Here's how the part is built. I have some questions about the finished solid (model axes, mm). A direction names the side the tool comes from. Give positions to 0.01 mm unless a question says otherwise; leave off trailing zeros. Write each loop counter-clockwise with the first axis right and the second up, starting at its lowest first coordinate (ties: lowest second). Pieces come first, ordered by that corner, then holes. Notation, with made-up numbers: (69.5, 80) -> (121.5, 80) arc R24 ccw to (121.5, 107) -> close; hole circle Ø5 at (24, 12.25). An arc over 180 degrees is marked (long way). Use CSV: the item, a comma, the result in double quotes. Start each with the question number.
(1) If we mould it in two halves opening along Y, with no side actions, what happens to faces 1 (the flat face through (60, 18, 8)), 2 (the flat face through (64, 18, 15))? For each: pulls with the +Y half, pulls with the -Y half, needs draft (parallel to the pull), parting line crosses it, or undercut.
(2) Suppose I cut it at C-C on z = 11.75. List the corners of the cut face in (x, y) for me, plus the area to 3 significant figures.
(3) Suppose I cut it at D-D on x = 9. List the corners of the cut face in (y, z) for me, plus the area to 3 significant figures.
(4) For pin 1 Ø4.5 at (x, y) = (31, 25.5) entering from +Z; pin 2 Ø2.5 at (x, y) = (3, 17.5) entering from +Z (1 decimal), each with a flat end and sliding along its axis, tell me the tip position at first contact or that it passes through.
(5) Suppose I cut it at A-A on x = 31. List the corners of the cut face in (y, z) for me.
(6) Suppose I cut it at B-B on y = 25.5. List the corners of the cut face in (x, z) for me (3 decimals).
(7) Which directions (+Z, -Z, +X, -X, +Y, -Y) give clear straight access to the entire face, cutting with the end or side of a thin tool? Please do faces 3 (the flat face through (31, 17, 0)), 4 (the flat face through (30, 2, 6)), 5 (the cylindrical face through (71, 3, 14)).
(8) I need wall thicknesses on L1, parallel to X at y = 19.5, z = 12.25; L2, parallel to X at y = 13.5, z = 8.25; L3, parallel to Y at x = 31, z = 2.35. Which ranges of each line are inside material? Lowest first, please. Write a range as [from, to].
from build123d import *

# Parameters (mm, degrees)
SKETCH_W             = 80
SKETCH_H             = 35
PAD_DEPTH            = 15
SKETCH001_R          = 2.5
POCKET_DEPTH         = 14
SKETCH002_W          = 61
SKETCH002_H          = 33.5
POCKET001_DEPTH      = 5
SKETCH003_R          = 1.5
POCKET002_DEPTH      = 5
SKETCH004_R          = 4
PAD001_DEPTH         = 5
SKETCH005_R          = 2
POCKET003_DEPTH      = 5
SKETCH006_W          = 16.25
SKETCH006_H          = 33
POCKET004_DEPTH      = 13
POCKET005_DEPTH      = 15.001
SKETCH008_R          = 2
POCKET006_DEPTH      = 5.001
POCKET006_DEPTH_BACK = -10.001
SKETCH009_R          = 2
POCKET007_DEPTH      = 2.75


with BuildPart() as part:
    # Sketch → Pad (new body)
    with BuildSketch(Plane.XY):
        with Locations((40, 17.5)):
            Rectangle(SKETCH_W, SKETCH_H)
    extrude(amount=PAD_DEPTH)

    # Sketch001 (on Face6 of Pad) → Pocket (cut)
    with BuildSketch(Plane.XY.offset(15)):
        with BuildLine():
            Line((2, 33), (60, 33))
            Line((60, 33), (60, 2))
            Line((53.5, 2), (60, 2))
            ThreePointArc((53.5, 2), (52, 6.5), (50.5, 2))
            Line((10.5, 2), (50.5, 2))
            ThreePointArc((10.5, 2), (9, 6.5), (7.5, 2))
            Line((2, 2), (7.5, 2))
            Line((2, 2), (2, 33))
        make_face()
        with Locations((9, 29)):
            Circle(SKETCH001_R, mode=Mode.SUBTRACT)
        with Locations((52, 29)):
            Circle(SKETCH001_R, mode=Mode.SUBTRACT)
    extrude(amount=-POCKET_DEPTH, mode=Mode.SUBTRACT)

    # Sketch002 (on Face5 of Pocket) → Pocket001 (cut)
    with BuildSketch(Plane.XY.offset(15)):
        with Locations((31.25, 17.5)):
            Rectangle(SKETCH002_W, SKETCH002_H)
    extrude(amount=-POCKET001_DEPTH, mode=Mode.SUBTRACT)

    # Sketch003 (on Face24 of Pocket001) → Pocket002 (cut)
    with BuildSketch(Plane.XY.offset(10)):
        with Locations((9, 29)):
            Circle(SKETCH003_R)
        with Locations((9, 4)):
            Circle(SKETCH003_R)
        with Locations((52, 29)):
            Circle(SKETCH003_R)
        with Locations((52, 4)):
            Circle(SKETCH003_R)
    extrude(amount=-POCKET002_DEPTH, mode=Mode.SUBTRACT)

    # Sketch004 (on Face4 of Pocket002) → Pad001 (join)
    with BuildSketch(Plane(origin=(0, 0, 0), x_dir=(1, 0, 0), z_dir=(0, 0, -1))):
        with Locations((31, -9.5)):
            Circle(SKETCH004_R)
        with Locations((31, -25.5)):
            Circle(SKETCH004_R)
    extrude(amount=-PAD001_DEPTH)

    # Sketch005 (on Face4 of Pad001) → Pocket003 (cut)
    with BuildSketch(Plane(origin=(0, 0, 0), x_dir=(1, 0, 0), z_dir=(0, 0, -1))):
        with Locations((31, -9.5)):
            Circle(SKETCH005_R)
        with Locations((31, -25.5)):
            Circle(SKETCH005_R)
    extrude(amount=-POCKET003_DEPTH, mode=Mode.SUBTRACT)

    # Sketch006 (on Face4 of Pocket003) → Pocket004 (cut)
    with BuildSketch(Plane(origin=(0, 0, 0), x_dir=(1, 0, 0), z_dir=(0, 0, -1))):
        with Locations((70.875, -17.5)):
            Rectangle(SKETCH006_W, SKETCH006_H)
    extrude(amount=-POCKET004_DEPTH, mode=Mode.SUBTRACT)

    # Sketch007 (on Face5 of Pocket004) → Pocket005 (cut, through all)
    with BuildSketch(Plane.XY.offset(15)):
        with BuildLine():
            Line((65.375, 28.397916), (65.375, 23.602084))
            ThreePointArc((65.375, 23.602084), (70.875, 20), (76.375, 23.602084))
            Line((76.375, 28.397916), (76.375, 23.602084))
            ThreePointArc((76.375, 28.397916), (70.875, 32), (65.375, 28.397916))
        make_face()
        with BuildLine():
            Line((65.375, 11.397916), (65.375, 6.602084))
            ThreePointArc((65.375, 6.602084), (70.875, 3), (76.375, 6.602084))
            Line((76.375, 11.397916), (76.375, 6.602084))
            ThreePointArc((76.375, 11.397916), (70.875, 15), (65.375, 11.397916))
        make_face()
    extrude(amount=-POCKET005_DEPTH, mode=Mode.SUBTRACT)

    # Sketch008 (on Face43 of Pocket005) → Pocket006 (cut, two sides)
    with BuildSketch(Plane.XY.offset(5)) as pocket006_sk:
        with Locations((3, 17.5)):
            Circle(SKETCH008_R)
    extrude(amount=-POCKET006_DEPTH, mode=Mode.SUBTRACT)
    extrude(pocket006_sk.sketch, amount=-POCKET006_DEPTH_BACK, mode=Mode.SUBTRACT)

    # Sketch009 (on Face37 of Pocket006) → Pocket007 (cut)
    with BuildSketch(Plane(origin=(60, 0, 0), x_dir=(0, -1, 0), z_dir=(-1, 0, 0))):
        with Locations((-17.5, 5.5)):
            Circle(SKETCH009_R)
    extrude(amount=-POCKET007_DEPTH, mode=Mode.SUBTRACT)


solid = part.part
Geometry says:
1,face 1,"undercut"
1,face 2,"needs draft"
2,outline,"(0, 0) -> (80, 0) -> (80, 35) -> (0, 35) -> close; hole (0.75, 0.75) -> (61.75, 0.75) -> (61.75, 34.25) -> (0.75, 34.25) -> close; hole (62.75, 1) -> (79, 1) -> (79, 34) -> (62.75, 34) -> close"
2,area,"220 mm²"
3,outline,"(0, 0) -> (35, 0) -> (35, 15) -> (34.25, 15) -> (34.25, 10) -> (33, 10) -> (33, 1) -> (31.5, 1) -> (31.5, 10) -> (30.5, 10) -> (30.5, 5) -> (27.5, 5) -> (27.5, 10) -> (26.5, 10) -> (26.5, 1) -> (6.5, 1) -> (6.5, 10) -> (5.5, 10) -> (5.5, 5) -> (2.5, 5) -> (2.5, 10) -> (0.75, 10) -> (0.75, 15) -> (0, 15) -> close"
3,area,"134 mm²"
4,pin 1,"z = 5"
4,pin 2,"through"
5,outline,"(0, 0) -> (7.5, 0) -> (7.5, 5) -> (5.5, 5) -> (5.5, 1) -> (2, 1) -> (2, 10) -> (0.75, 10) -> (0.75, 15) -> (0, 15) -> close; (11.5, 0) -> (23.5, 0) -> (23.5, 5) -> (21.5, 5) -> (21.5, 1) -> (13.5, 1) -> (13.5, 5) -> (11.5, 5) -> close; (27.5, 0) -> (35, 0) -> (35, 15) -> (34.25, 15) -> (34.25, 10) -> (33, 10) -> (33, 1) -> (29.5, 1) -> (29.5, 5) -> (27.5, 5) -> close"
6,outline,"(0, 0) -> (29, 0) -> (29, 5) -> (27, 5) -> (27, 1) -> (2, 1) -> (2, 10) -> (0.75, 10) -> (0.75, 15) -> (0, 15) -> close; (33, 0) -> (62.75, 0) -> (62.75, 13) -> (65.375, 13) -> (65.375, 15) -> (61.75, 15) -> (61.75, 10) -> (60, 10) -> (60, 1) -> (35, 1) -> (35, 5) -> (33, 5) -> close; (76.375, 13) -> (79, 13) -> (79, 0) -> (80, 0) -> (80, 15) -> (76.375, 15) -> close"
7,face 3,"-Z, +X, -X, +Y, -Y"
7,face 4,"+Z"
7,face 5,"+Z, -Z"
8,L1,"[0, 0.75], [61.75, 62.75], [79, 80]"
8,L2,"[0, 2], [60, 62.75], [79, 80]"
8,L3,"[0, 2], [5.5, 7.5], [11.5, 13.5], [21.5, 23.5], [27.5, 29.5], [33, 35]"
